Job drawing, mm, ordinate dimensions from the low corner. One solid piece. Give positions to 0.01 mm unless a question says otherwise; leave off trailing zeros. Loops run counter-clockwise (first coordinate to the right, second up) from the corner with the lowest first, then second, coordinate; pieces in that order, holes last. Notation, with made-up numbers: M -29.5,16.25 L -5.5,16.25 A25 cw -5.5,48.25 Z; hole C 14,-2 d8. An arc over 180 degrees is marked long. Answer in a Markdown table with one row per item.
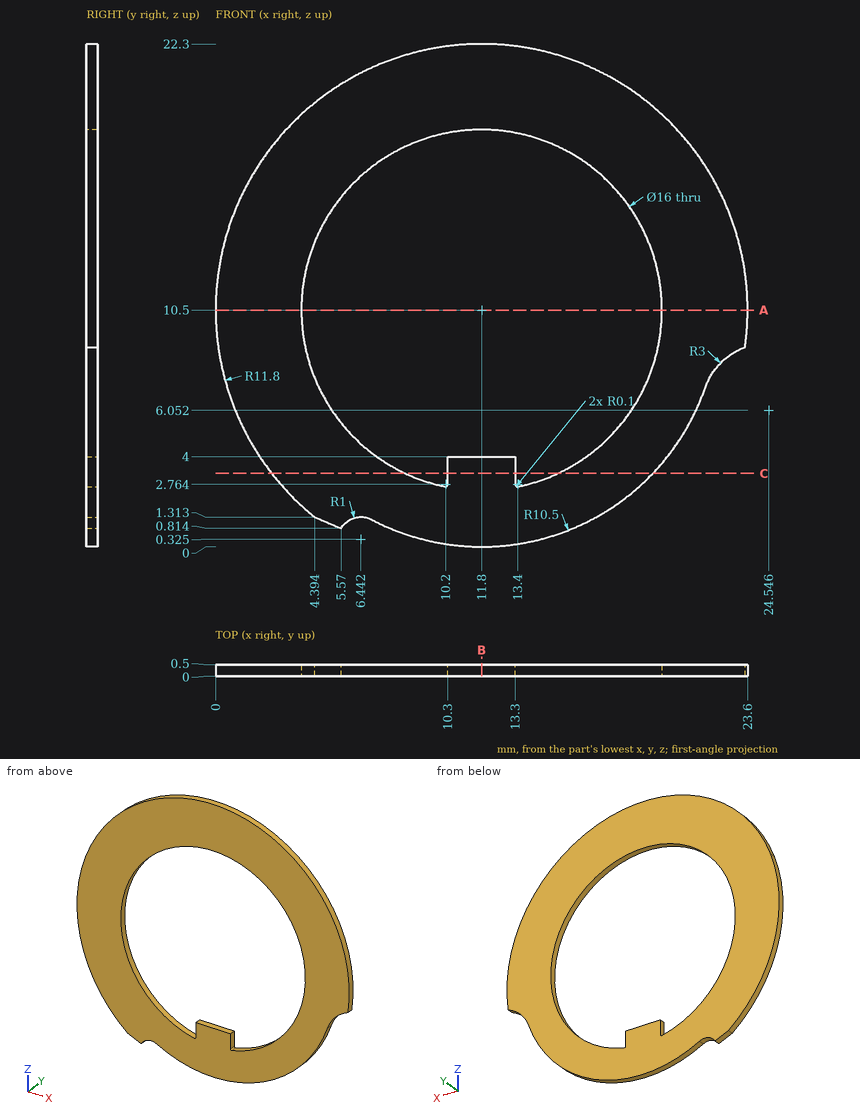
(1) Saw through at B-B (x = 11.8). Write the cut outline in (y, z).
Recorded:
| item | result |
|---|---|
| outline | M 0,0 L 0.5,0 L 0.5,4 L 0,4 Z; M 0,18.5 L 0.5,18.5 L 0.5,22.3 L 0,22.3 Z |
(2) Saw through at C-C (z = 3.25). Write the cut outline in (x, y) (1 decimal).
Recorded:
| item | result |
|---|---|
| outline | M 2.5,0 L 8.4,0 L 8.4,0.5 L 2.5,0.5 Z; M 10.3,0 L 13.3,0 L 13.3,0.5 L 10.3,0.5 Z; M 15.2,0 L 19.4,0 L 19.4,0.5 L 15.2,0.5 Z |
(3) Drill centre lines: line 1 along X through (y, z) = (0.1, 10.75); line 2 along X through (y, z) = (0.3, 14) (1 decimal); line 3 along Z through (x, y) = (17.5, 0.35) (1 decimal). Where is each one in solid material? Low to high.
Recorded:
| item | result |
|---|---|
| line 1 | x = 0 to 3.8, 19.8 to 23.6 |
| line 2 | x = 0.5 to 4.6, 19 to 23.1 |
| line 3 | z = 1.7 to 4.9, 16.1 to 20.8 |
(4) Saw through at A-A (z = 10.5). Write the cut outline in (x, y).
Recorded:
| item | result |
|---|---|
| outline | M 0,0 L 3.8,0 L 3.8,0.5 L 0,0.5 Z; M 19.8,0 L 23.6,0 L 23.6,0.5 L 19.8,0.5 Z |
